Geometry check sheet. Reference: the model listing, model coordinates, mm. A direction names the side the tool comes from. Round coordinates to 2 decimals unless told otherwise and drop trailing zeros. Loops run counter-clockwise (first coordinate to the right, second up) from the corner with the lowest first, then second, coordinate; pieces in that order, holes last.
```python
from build123d import *

# Parameters (mm, degrees)
SKETCH1_W           = 25
SKETCH1_H           = 20
BOSS_EXTRUDE1_DEPTH = 2.5
SKETCH4_R           = 10
BOSS_EXTRUDE3_DEPTH = 1
SKETCH5_R           = 4.9365
BOSS_EXTRUDE4_DEPTH = 20
SKETCH6_R           = 1.627
BOSS_EXTRUDE5_DEPTH = 2.5


with BuildPart() as part:
    # Sketch1 → Boss-Extrude1 (new body)
    with BuildSketch(Plane(origin=(0, 0, 0), x_dir=(1, 0, 0), z_dir=(0, 1, 0))):
        Rectangle(SKETCH1_W, SKETCH1_H)
    extrude(amount=BOSS_EXTRUDE1_DEPTH)

    # Sketch4 → Boss-Extrude3 (add)
    with BuildSketch(Plane.XZ):
        with Locations(Location((0, 0, 0), (0, 0, 270))):
            Circle(SKETCH4_R)
    extrude(amount=BOSS_EXTRUDE3_DEPTH)

    # Sketch5 → Boss-Extrude4 (add)
    with BuildSketch(Plane.XZ.offset(1)):
        with Locations(Location((0, 0, 0), (0, 0, 270))):
            Circle(SKETCH5_R)
    extrude(amount=BOSS_EXTRUDE4_DEPTH)

    # Sketch6 → Boss-Extrude5 (add)
    with BuildSketch(Plane(origin=(0, 0, -10), x_dir=(-1, 0, 0), z_dir=(0, 0, -1))):
        with BuildLine():
            Line((-12.150452519, 2.5), (12.150452519, 2.5))
            Line((12.150452519, 2.5), (5.334920531, 51.245394823))
            ThreePointArc((5.334920531, 51.245394823), (0, 55.886742106), (-5.334920531, 51.245394823))
            Line((-5.334920531, 51.245394823), (-12.150452519, 2.5))
        make_face()
        with Locations((0, 50.5)):
            Circle(SKETCH6_R, mode=Mode.SUBTRACT)
    boss_extrude5 = extrude(amount=-BOSS_EXTRUDE5_DEPTH)

    # Mirror2: Boss-Extrude5 across plane
    add(boss_extrude5.mirror(Plane(origin=(0, 0, 0), x_dir=(1, 0, 0), z_dir=(0, 0, -1))))


solid = part.part
```
1) Sectioned sample at C-C, the plane x = 7.5. Record the cut outline in (y, z).
Report:
outline: (-1, -6.61) - (0, -6.61) - (0, -10) - (35.76, -10) - (35.76, -7.5) - (2.5, -7.5) - (2.5, 7.5) - (35.76, 7.5) - (35.76, 10) - (0, 10) - (0, 6.61) - (-1, 6.61) - close
2) Mould release check, pull along Y, two halves, no side actions. Record for faces 5 (the face through (-12.5, 1, 0)), 6 (the face through (0.212, 52.113, -8.768)), 7 (the face through (-8.79, 26.53, -8.77)): +Y half, -Y half, draft (parallel to the pull), parting line (faces both ways), or undercut.
Report:
face 5: draft
face 6: undercut
face 7: +Y half
3) Access from +Z, -Z, +X, -X, +Y, -Y to the whole of each face (thin tool, end or side, straight path). Record for faces 1 (the face through (12.5, 1, 0)), 2 (the face through (-11, 0, 0)), 3 (the face through (-9.76, -0.49, 2.17)), 4 (the face through (0, 24, 7.5)).
Report:
face 1: +Z, -Z, +X, +Y, -Y
face 2: -X, -Y
face 3: -Y
face 4: +X, -X, +Y
4) Scan lines: line 1 along Z through (x, y) = (1.5, 25.5); line 2 along Y through (x, z) = (7.25, -6.5); line 3 along Y through (x, z) = (-1, 1). Record each from-to range of solid material in increasing order.
Report:
line 1: z = -10 to -7.5, 7.5 to 10
line 2: y = -1 to 2.5
line 3: y = -21 to 2.5
5) Gauge pin test, flat ends, axial feed: pin 1 (1 mm diameter, centred on x = 7.5, z = -3.5, fed in from -Y); pin 2 (10 mm diameter, centred on y = 32.5, z = -7.5, fed in from +X) (3 decimals); pin 3 (6 mm diameter, centred on x = -1.5, z = -2.5, fed in from +Y). Record the tip position at first contact, or that the pin passes through.
Report:
pin 1: stops at y = -1
pin 2: stops at x = 8.655
pin 3: stops at y = 2.5
6) Sectioned sample at D-D, the plane y = 5. Record the cut outline in (x, z).
Report:
outline: (-11.8, -10) - (11.8, -10) - (11.8, -7.5) - (-11.8, -7.5) - close; (-11.8, 7.5) - (11.8, 7.5) - (11.8, 10) - (-11.8, 10) - close
7) Sectioned sample at B-B, the plane z = 0. Record the cut outline in (x, y), then the cut area to 3 significant figures.
Report:
outline: (-12.5, 0) - (-10, 0) - (-10, -1) - (-4.94, -1) - (-4.94, -21) - (4.94, -21) - (4.94, -1) - (10, -1) - (10, 0) - (12.5, 0) - (12.5, 2.5) - (-12.5, 2.5) - close
area: 280 mm2
8) Sectioned sample at A-A, the plane y = 50.5. Record the cut outline in (x, z), then the cut area to 3 significant figures.
Report:
outline: (-5.44, -10) - (-1.63, -10) - (-1.63, -7.5) - (-5.44, -7.5) - close; (-5.44, 7.5) - (-1.63, 7.5) - (-1.63, 10) - (-5.44, 10) - close; (1.63, -10) - (5.44, -10) - (5.44, -7.5) - (1.63, -7.5) - close; (1.63, 7.5) - (5.44, 7.5) - (5.44, 10) - (1.63, 10) - close
area: 38.1 mm2
